```python
from build123d import *

# Parameters (mm, degrees)
F1_DEPTH = 1
F2_DEPTH = 60
F2_TAPER = 3
F3_DEPTH = 60
F3_TAPER = 3
F5_DEPTH = 0.7


with BuildPart() as f1:
    # F0 (on Top) → F1 (new body)
    with BuildSketch(Plane.XY):
        with BuildLine():
            Line((39.2, 55), (-39.2, 55))
            ThreePointArc((-39.2, 55), (-50.3722871427, 50.3722871427), (-55, 39.2))
            Line((-55, 39.2), (-55, -39.2))
            ThreePointArc((-55, -39.2), (-50.3722871427, -50.3722871427), (-39.2, -55))
            Line((-39.2, -55), (39.2, -55))
            ThreePointArc((39.2, -55), (50.3722871427, -50.3722871427), (55, -39.2))
            Line((55, -39.2), (55, 39.2))
            ThreePointArc((55, 39.2), (50.3722871427, 50.3722871427), (39.2, 55))
        make_face()
        with BuildLine():
            ThreePointArc((-53.8, 38.8), (-49.4066017178, 49.4066017178), (-38.8, 53.8))
            Line((-38.8, 53.8), (38.8, 53.8))
            ThreePointArc((38.8, 53.8), (49.4066017178, 49.4066017178), (53.8, 38.8))
            Line((53.8, 38.8), (53.8, -38.8))
            ThreePointArc((53.8, -38.8), (49.4066017178, -49.4066017178), (38.8, -53.8))
            Line((38.8, -53.8), (-38.8, -53.8))
            ThreePointArc((-38.8, -53.8), (-49.4066017178, -49.4066017178), (-53.8, -38.8))
            Line((-53.8, -38.8), (-53.8, 38.8))
        make_face(mode=Mode.SUBTRACT)
    extrude(amount=F1_DEPTH)

    # F0 (on Top) → F2 (join)
    with BuildSketch(Plane.XY):
        with BuildLine():
            Line((39.2, 55), (-39.2, 55))
            ThreePointArc((-39.2, 55), (-50.3722871427, 50.3722871427), (-55, 39.2))
            Line((-55, 39.2), (-55, -39.2))
            ThreePointArc((-55, -39.2), (-50.3722871427, -50.3722871427), (-39.2, -55))
            Line((-39.2, -55), (39.2, -55))
            ThreePointArc((39.2, -55), (50.3722871427, -50.3722871427), (55, -39.2))
            Line((55, -39.2), (55, 39.2))
            ThreePointArc((55, 39.2), (50.3722871427, 50.3722871427), (39.2, 55))
        make_face()
        with BuildLine():
            ThreePointArc((-53.8, 38.8), (-49.4066017178, 49.4066017178), (-38.8, 53.8))
            Line((-38.8, 53.8), (38.8, 53.8))
            ThreePointArc((38.8, 53.8), (49.4066017178, 49.4066017178), (53.8, 38.8))
            Line((53.8, 38.8), (53.8, -38.8))
            ThreePointArc((53.8, -38.8), (49.4066017178, -49.4066017178), (38.8, -53.8))
            Line((38.8, -53.8), (-38.8, -53.8))
            ThreePointArc((-38.8, -53.8), (-49.4066017178, -49.4066017178), (-53.8, -38.8))
            Line((-53.8, -38.8), (-53.8, 38.8))
        make_face(mode=Mode.SUBTRACT)
        with BuildLine():
            Line((38.8, 53.8), (-38.8, 53.8))
            ThreePointArc((-38.8, 53.8), (-49.4066017178, 49.4066017178), (-53.8, 38.8))
            Line((-53.8, 38.8), (-53.8, -38.8))
            ThreePointArc((-53.8, -38.8), (-49.4066017178, -49.4066017178), (-38.8, -53.8))
            Line((-38.8, -53.8), (38.8, -53.8))
            ThreePointArc((38.8, -53.8), (49.4066017178, -49.4066017178), (53.8, -38.8))
            Line((53.8, -38.8), (53.8, 38.8))
            ThreePointArc((53.8, 38.8), (49.4066017178, 49.4066017178), (38.8, 53.8))
        make_face()
    extrude(amount=-F2_DEPTH, taper=F2_TAPER)

    # F0 (on Top) → F3 (cut)
    with BuildSketch(Plane.XY):
        with BuildLine():
            Line((38.8, 53.8), (-38.8, 53.8))
            ThreePointArc((-38.8, 53.8), (-49.4066017178, 49.4066017178), (-53.8, 38.8))
            Line((-53.8, 38.8), (-53.8, -38.8))
            ThreePointArc((-53.8, -38.8), (-49.4066017178, -49.4066017178), (-38.8, -53.8))
            Line((-38.8, -53.8), (38.8, -53.8))
            ThreePointArc((38.8, -53.8), (49.4066017178, -49.4066017178), (53.8, -38.8))
            Line((53.8, -38.8), (53.8, 38.8))
            ThreePointArc((53.8, 38.8), (49.4066017178, 49.4066017178), (38.8, 53.8))
        make_face()
    extrude(amount=-F3_DEPTH, taper=F3_TAPER, mode=Mode.SUBTRACT)

    # F4 (on face) → F5 (join)
    with BuildSketch(Plane(origin=(0, 0, -60), x_dir=(1, 0, 0), z_dir=(0, 0, -1))):
        with BuildLine():
            ThreePointArc((39.2, -51.855533243), (48.1488133757, -48.1488133757), (51.855533243, -39.2))
            Line((51.855533243, -39.2), (51.855533243, 39.2))
            ThreePointArc((51.855533243, 39.2), (48.1488133757, 48.1488133757), (39.2, 51.855533243))
            Line((39.2, 51.855533243), (-39.2, 51.855533243))
            ThreePointArc((-39.2, 51.855533243), (-48.1488133757, 48.1488133757), (-51.855533243, 39.2))
            Line((-51.855533243, 39.2), (-51.855533243, -39.2))
            ThreePointArc((-51.855533243, -39.2), (-48.1488133757, -48.1488133757), (-39.2, -51.855533243))
            Line((-39.2, -51.855533243), (39.2, -51.855533243))
        make_face()
        with BuildLine():
            ThreePointArc((50.655533243, -38.8), (47.1831279507, -47.1831279507), (38.8, -50.655533243))
            Line((38.8, -50.655533243), (-38.8, -50.655533243))
            ThreePointArc((-38.8, -50.655533243), (-47.1831279507, -47.1831279507), (-50.655533243, -38.8))
            Line((-50.655533243, -38.8), (-50.655533243, 38.8))
            ThreePointArc((-50.655533243, 38.8), (-47.1831279507, 47.1831279507), (-38.8, 50.655533243))
            Line((-38.8, 50.655533243), (38.8, 50.655533243))
            ThreePointArc((38.8, 50.655533243), (47.1831279507, 47.1831279507), (50.655533243, 38.8))
            Line((50.655533243, 38.8), (50.655533243, -38.8))
        make_face(mode=Mode.SUBTRACT)
        with BuildLine():
            Line((-38.8, -50.655533243), (38.8, -50.655533243))
            ThreePointArc((38.8, -50.655533243), (47.1831279507, -47.1831279507), (50.655533243, -38.8))
            Line((50.655533243, -38.8), (50.655533243, 38.8))
            ThreePointArc((50.655533243, 38.8), (47.1831279507, 47.1831279507), (38.8, 50.655533243))
            Line((38.8, 50.655533243), (-38.8, 50.655533243))
            ThreePointArc((-38.8, 50.655533243), (-47.1831279507, 47.1831279507), (-50.655533243, 38.8))
            Line((-50.655533243, 38.8), (-50.655533243, -38.8))
            ThreePointArc((-50.655533243, -38.8), (-47.1831279507, -47.1831279507), (-38.8, -50.655533243))
        make_face()
    extrude(amount=F5_DEPTH)


solid = f1.part
```
Source: CAD feature listing. Evaluate the final solid. Frame: model axes, mm. A direction names the side the tool comes from. Give positions to 0.01 mm unless a question says otherwise; leave off trailing zeros.
(1) Pull-direction query (X, two-part tool) for faces 6 (the face through (-49.29, -49.52, 0.49)), 7 (the face through (49.355, 49.134, -30.42)), 8 (the face through (-1, -1, -60.7)), 9 (the face through (-0.543, -52.206, -30.42)); classes: +X half, -X half, draft (parallel to the pull), parting line (faces both ways), or undercut.
(2) Access query for faces 1 (the face through (-48.05, -48.247, -60.345)), 2 (the face through (48.247, -48.05, -60.345)), 3 (the face through (50.249, -50.494, 0.493)), 4 (the face through (48.174, -48.383, -30.42)), 5 (the face through (-50.249, 50.494, 0.493)). Directions: +Z, -Z, +X, -X, +Y, -Y. A direction counts if a zero-diameter tool reaches every point of the face in a straight line with its end or side. Return the directions, or none.
(3) Material intervals for line 1 along Z through (x, y) = (-34, 20.5); line 2 along Y through (x, z) = (31, -36.5); line 3 along X through (y, z) = (5.5, -32), sorted ascending.
(4) Contact query for flat-ended pins moving along their axis: P1, Ø0.6, axis at x = -3, z = -60, coming from the +Y side; P2, Ø0.6, axis at y = 12.5, z = -60.5, coming from the -X side; P3, Ø1.5, axis at x = -33, z = -18, coming from the +Y side. Output: stop coordinate, or through.
Outcome:
1. face 6: undercut
1. face 7: +X half
1. face 8: draft
1. face 9: undercut
2. face 1: -Z, -X, -Y
2. face 2: -Z, +X, -Y
2. face 3: +Z, -Z, +X, -Y
2. face 4: +Z
2. face 5: +Z, -Z, -X, +Y
3. line 1: z = -60.7 to -60
3. line 2: y = -53.09 to -51.89, 51.89 to 53.09
3. line 3: x = -53.32 to -52.12, 52.12 to 53.32
4. P1: stops at y = 51.87
4. P2: stops at x = -51.86
4. P3: stops at y = 54.1
